Check sheet for the modelled part. Datum: model origin and axes. Units: mm. Face numbers are marked on the shaded views. Round coordinates to 2 decimals unless told otherwise and drop trailing zeros. Put each result on its own line as item: value. Start each with the question number.
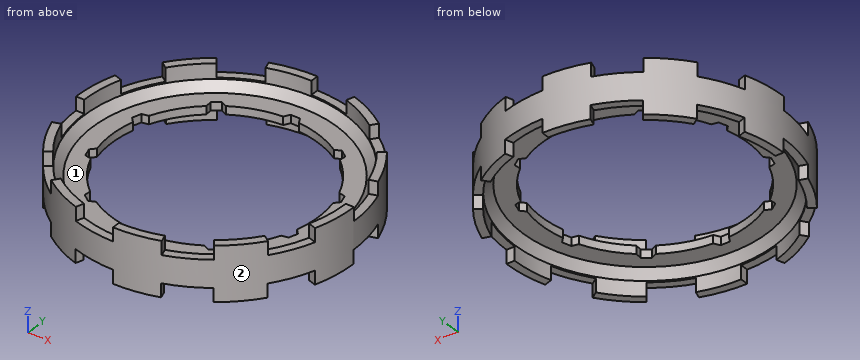
```python
from build123d import *

# Parameters (mm, degrees)
F0_R      = 51
F0_R_2    = 48
F1_DEPTH  = 10
F0_R_3    = 38
F2_DEPTH  = 1.5
F5_DEPTH  = 25
F8_DEPTH  = 25
F11_DEPTH = 25
F12_SIZE  = 3


with BuildPart() as f1:
    # F0 (on Top) → F1 (new body, symmetric)
    with BuildSketch(Plane.XY):
        Circle(F0_R)
        Circle(F0_R_2, mode=Mode.SUBTRACT)
    extrude(amount=F1_DEPTH, both=True)

    # F0 (on Top) → F2 (join, symmetric)
    with BuildSketch(Plane.XY):
        Circle(F0_R_2)
        Circle(F0_R_3, mode=Mode.SUBTRACT)
    extrude(amount=F2_DEPTH, both=True)

    # F4 (on offset) → F5 (cut)
    with BuildSketch(Plane.XY.offset(15)):
        Polygon((-1.690599, 40), (-4, 36), (4, 36), (1.690599, 40), align=None)
        Polygon((-17.924201, 31.475753), (-22.143687, 33.354389), (-24.879133, 31.366971), (-24.396337, 26.773471), align=None)
        Polygon((-33.001967, 14.928838), (-37.519837, 13.968535), (-38.564684, 10.752825), (-35.474103, 7.320386), align=None)
        Polygon((-35.474103, -7.320386), (-38.564684, -10.752825), (-37.519837, -13.968535), (-33.001967, -14.928838), align=None)
        Polygon((-24.396337, -26.773471), (-24.879133, -31.366971), (-22.143687, -33.354389), (-17.924201, -31.475753), align=None)
        Polygon((-4, -36), (-1.690599, -40), (1.690599, -40), (4, -36), align=None)
        Polygon((17.924201, -31.475753), (22.143687, -33.354389), (24.879133, -31.366971), (24.396337, -26.773471), align=None)
        Polygon((33.001967, -14.928838), (37.519837, -13.968535), (38.564684, -10.752825), (35.474103, -7.320386), align=None)
        Polygon((35.474103, 7.320386), (38.564684, 10.752825), (37.519837, 13.968535), (33.001967, 14.928838), align=None)
        Polygon((24.396337, 26.773471), (24.879133, 31.366971), (22.143687, 33.354389), (17.924201, 31.475753), align=None)
    extrude(amount=-F5_DEPTH, mode=Mode.SUBTRACT)

    # F7 (on offset) → F8 (cut)
    with BuildSketch(Plane.XY.offset(30)):
        with BuildLine():
            Line((0, 55.1512), (0, 35.000008))
            ThreePointArc((0, 35.000008), (5.367163, 34.584221), (10.606253, 33.346784))
            Line((10.606253, 33.346784), (16.739279, 52.542006))
            ThreePointArc((16.739279, 52.542006), (8.470705, 54.494987), (0, 55.1512))
        make_face()
        with BuildLine():
            Line((-32.401203, 44.569659), (-20.556629, 28.267002))
            ThreePointArc((-20.556629, 28.267002), (-15.97011, 31.085363), (-11.004249, 33.163715))
            Line((-11.004249, 33.163715), (-17.325195, 52.297878))
            ThreePointArc((-17.325195, 52.297878), (-25.162546, 49.017727), (-32.401203, 44.569659))
        make_face()
        with BuildLine():
            Line((-52.394652, 16.964063), (-33.229729, 10.737002))
            ThreePointArc((-33.229729, 10.737002), (-31.175748, 15.712992), (-28.379908, 20.313274))
            Line((-28.379908, 20.313274), (-44.740439, 32.077778))
            ThreePointArc((-44.740439, 32.077778), (-49.152965, 24.817401), (-52.394652, 16.964063))
        make_face()
        with BuildLine():
            Line((-52.343531, -17.121188), (-33.178608, -10.894127))
            ThreePointArc((-33.178608, -10.894127), (-34.441716, -5.661167), (-34.883811, -0.296107))
            Line((-34.883811, -0.296107), (-55.034761, -0.394902))
            ThreePointArc((-55.034761, -0.394902), (-54.337027, -8.862288), (-52.343531, -17.121188))
        make_face()
        with BuildLine():
            Line((-32.267365, -44.666687), (-20.422791, -28.36403))
            ThreePointArc((-20.422791, -28.36403), (-24.520524, -24.872912), (-28.031689, -20.792345))
            Line((-28.031689, -20.792345), (-44.27608, -32.716703))
            ThreePointArc((-44.27608, -32.716703), (-38.734596, -39.156844), (-32.267365, -44.666687))
        make_face()
        with BuildLine():
            Line((0.165433, -55.150989), (0.165433, -34.999797))
            ThreePointArc((0.165433, -34.999797), (-5.20173, -34.58401), (-10.44082, -33.346573))
            Line((-10.44082, -33.346573), (-16.573846, -52.541795))
            ThreePointArc((-16.573846, -52.541795), (-8.305272, -54.494776), (0.165433, -55.150989))
        make_face()
        with BuildLine():
            Line((32.566636, -44.569448), (20.722062, -28.266791))
            ThreePointArc((20.722062, -28.266791), (16.135543, -31.085152), (11.169682, -33.163504))
            Line((11.169682, -33.163504), (17.490629, -52.297667))
            ThreePointArc((17.490629, -52.297667), (25.327979, -49.017516), (32.566636, -44.569448))
        make_face()
        with BuildLine():
            Line((52.560085, -16.963852), (33.395162, -10.736791))
            ThreePointArc((33.395162, -10.736791), (31.341182, -15.712781), (28.545341, -20.313063))
            Line((28.545341, -20.313063), (44.905873, -32.077567))
            ThreePointArc((44.905873, -32.077567), (49.318398, -24.81719), (52.560085, -16.963852))
        make_face()
        with BuildLine():
            Line((52.508964, 17.121399), (33.344041, 10.894338))
            ThreePointArc((33.344041, 10.894338), (34.607149, 5.661378), (35.049244, 0.296318))
            Line((35.049244, 0.296318), (55.200194, 0.395113))
            ThreePointArc((55.200194, 0.395113), (54.50246, 8.862499), (52.508964, 17.121399))
        make_face()
        with BuildLine():
            Line((32.432798, 44.666898), (20.588224, 28.364241))
            ThreePointArc((20.588224, 28.364241), (24.685957, 24.873123), (28.197122, 20.792556))
            Line((28.197122, 20.792556), (44.441513, 32.716914))
            ThreePointArc((44.441513, 32.716914), (38.900029, 39.157055), (32.432798, 44.666898))
        make_face()
    extrude(amount=-F8_DEPTH, mode=Mode.SUBTRACT)

    # F10 (on offset) → F11 (cut)
    with BuildSketch(Plane.XY.offset(-30)):
        with BuildLine():
            Line((0.082717, 55.000105), (0.082717, 35.346372))
            ThreePointArc((0.082717, 35.346372), (5.555695, 34.920086), (10.896661, 33.651511))
            Line((10.896661, 33.651511), (16.909585, 52.362845))
            ThreePointArc((16.909585, 52.362845), (8.598858, 54.336791), (0.082717, 55.000105))
        make_face()
        with BuildLine():
            Line((-32.245472, 44.49604), (-20.693297, 28.595835))
            ThreePointArc((-20.693297, 28.595835), (-16.015001, 31.467899), (-10.948419, 33.580942))
            Line((-10.948419, 33.580942), (-17.082107, 52.253037))
            ThreePointArc((-17.082107, 52.253037), (-24.965883, 48.965069), (-32.245472, 44.49604))
        make_face()
        with BuildLine():
            Line((-52.225392, 16.99604), (-33.53358, 10.922702))
            ThreePointArc((-33.53358, 10.922702), (-31.436915, 15.996084), (-28.57998, 20.683634))
            Line((-28.57998, 20.683634), (-44.51742, 32.184385))
            ThreePointArc((-44.51742, 32.184385), (-48.962909, 24.890396), (-52.225392, 16.99604))
        make_face()
        with BuildLine():
            Line((-52.225392, -16.995829), (-33.53358, -10.922491))
            ThreePointArc((-33.53358, -10.922491), (-34.819402, -5.585651), (-35.263365, -0.114078))
            Line((-35.263365, -0.114078), (-54.916996, -0.177568))
            ThreePointArc((-54.916996, -0.177568), (-54.226174, -8.691522), (-52.225392, -16.995829))
        make_face()
        with BuildLine():
            Line((-32.245472, -44.495829), (-20.693297, -28.595624))
            ThreePointArc((-20.693297, -28.595624), (-24.870465, -25.033816), (-28.445749, -20.868177))
            Line((-28.445749, -20.868177), (-44.308552, -32.471656))
            ThreePointArc((-44.308552, -32.471656), (-38.745288, -38.953534), (-32.245472, -44.495829))
        make_face()
        with BuildLine():
            Line((0.082717, -54.999895), (0.082717, -35.346161))
            ThreePointArc((0.082717, -35.346161), (-5.390261, -34.919875), (-10.731228, -33.6513))
            Line((-10.731228, -33.6513), (-16.744152, -52.362634))
            ThreePointArc((-16.744152, -52.362634), (-8.433425, -54.33658), (0.082717, -54.999895))
        make_face()
        with BuildLine():
            Line((32.410905, -44.495829), (20.85873, -28.595624))
            ThreePointArc((20.85873, -28.595624), (16.180434, -31.467688), (11.113852, -33.580731))
            Line((11.113852, -33.580731), (17.24754, -52.252826))
            ThreePointArc((17.24754, -52.252826), (25.131316, -48.964858), (32.410905, -44.495829))
        make_face()
        with BuildLine():
            Line((52.390825, -16.995829), (33.699013, -10.922491))
            ThreePointArc((33.699013, -10.922491), (31.602348, -15.995873), (28.745413, -20.683423))
            Line((28.745413, -20.683423), (44.682853, -32.184174))
            ThreePointArc((44.682853, -32.184174), (49.128343, -24.890185), (52.390825, -16.995829))
        make_face()
        with BuildLine():
            Line((52.390825, 16.99604), (33.699013, 10.922702))
            ThreePointArc((33.699013, 10.922702), (34.984835, 5.585862), (35.428798, 0.114289))
            Line((35.428798, 0.114289), (55.08243, 0.177779))
            ThreePointArc((55.08243, 0.177779), (54.391607, 8.691733), (52.390825, 16.99604))
        make_face()
        with BuildLine():
            Line((32.410905, 44.49604), (20.85873, 28.595835))
            ThreePointArc((20.85873, 28.595835), (25.035898, 25.034027), (28.611182, 20.868388))
            Line((28.611182, 20.868388), (44.473985, 32.471867))
            ThreePointArc((44.473985, 32.471867), (38.910722, 38.953745), (32.410905, 44.49604))
        make_face()
    extrude(amount=F11_DEPTH, mode=Mode.SUBTRACT)

    # F12
    f12_edges = [f1.edges().sort_by_distance(p)[0] for p in [
        (-48, 0, 1.5),
        (-48, 0, -1.5),
    ]]
    chamfer(f12_edges, length=F12_SIZE)


solid = f1.part
```
Q1. Material ranges on line 1 (X direction, y = 0, z = 6.7); line 2 (Y direction, x = 0, z = -8.2); line 3 (Y direction, x = -2.5, z = -1), recorded low to high. Write a range as from..to.
Q2. Depth check by flat-ended pin: pin 1 Ø5.5 at (x, y) = (-5, -48) entering from +Z; pin 2 Ø2.5 at (x, y) = (-48, -8.5) entering from -Z; pin 3 Ø10 at (x, z) = (2.5, -4.5) entering from +Y; pin 4 Ø12 at (y, z) = (-23, 5.5) entering from +X. Enter the tip coordinate at first touch or a pass-through.
Q3. Cross-section at A-A on z = 7. State how many separate pieces and enclosed holes the cut face has, and give its area (3 significant figures).
Q4. Draft check along Y on the marked faces 1 and 2. Enter one of: +Y half, -Y half, draft (parallel to the pull), parting line (faces both ways), or undercut.
Answer list:
1. line 1: x = -51..-48, 48..51
1. line 2: y = 48..51
1. line 3: y = -50.94..-38.6, 38.6..50.94
2. pin 1: stops at z = 5
2. pin 2: stops at z = -5
2. pin 3: stops at y = 51
2. pin 4: stops at x = 48.08
3. separate pieces: 10
3. enclosed holes: 0
3. area: 475 mm2
4. face 1: undercut
4. face 2: parting line
